Autodesk Inventor part; units mm, degrees
ref_plane "YZ Plane" through (0, 0, 0) normal (1, 0, 0) x (0, 1, 0)
ref_plane "XZ Plane" through (0, 0, 0) normal (0, 1, 0) x (-1, 0, 0)
ref_plane "XY Plane" through (0, 0, 0) normal (0, 0, 1) x (1, 0, 0)
sketch "Sketch1" plane through (0, 0, 0) normal (0, 1, 0) x (-1, 0, 0)
  line L0 (29.75, 29.75) -> (-29.75, 29.75)
  line L1 (-29.75, 29.75) -> (-29.75, -29.75)
  line L2 (-29.75, -29.75) -> (29.75, -29.75)
  line L3 (29.75, -29.75) -> (29.75, 29.75)
  line L4 (29.75, 0) -> (-29.75, 0) construction
  line L5 (0, -29.75) -> (0, 29.75) construction
  circle A0 centre (-22.75, 22.75) radius 1.75
  circle A1 centre (-22.75, -22.75) radius 1.75
  circle A2 centre (22.75, -22.75) radius 1.75
  circle A3 centre (22.75, 22.75) radius 1.75
  circle A4 centre (-1, 0) radius 0.25
  circle A5 centre (1, 0) radius 0.25
  point P0 (0, 0)
  dimension "d0" = 59.5
  dimension "d3" = 3.5
  dimension "d4" = 7
  dimension "d5" = 7
  dimension "d10" = 1
  dimension "d11" = 0.5
extrude "Extrusion1" add sketch "Sketch1" along normal blind 5
sketch "Sketch3" plane through (0, 5, 0) normal (0, 1, 0) x (1, 0, 0)
  circle A0 centre (0, 0) radius 24.25
  circle A1 centre (0, 0) radius 21.25
  line L0 (29.75, 29.75) -> (-29.75, 29.75)
  dimension "d7" = 3
  dimension "d12" = 5.5
extrude "Extrusion2" add sketch "Sketch3" along normal blind 4
properties part number "Power_Meter_Adapter_Part2"
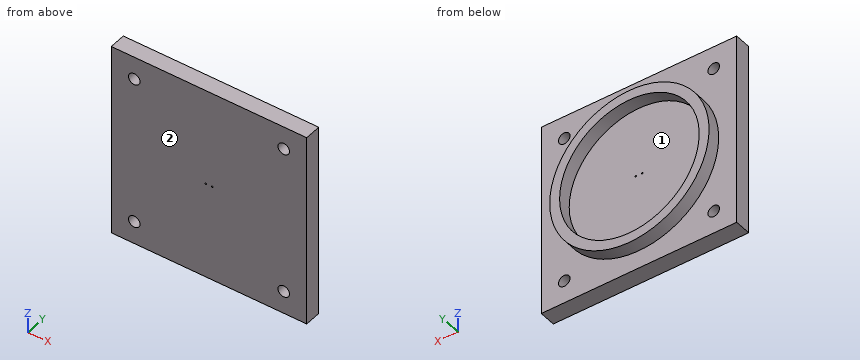
Check sheet for the modelled part. Datum: model origin and axes. Units: mm. Face numbers are marked on the shaded views. Coordinates: 2 decimals unless noted, no trailing zeros. Write each loop counter-clockwise with the first axis right and the second up, starting at its lowest first coordinate (ties: lowest second). Pieces come first, ordered by that corner, then holes.
Item 1: Mould release check, pull along Z, two halves, no side actions. Record for the marked faces 1 and 2: released by +Z, released by -Z, zero draft, split by the parting line, or undercut.
Numbers:
face 1: undercut
face 2: zero draft
Item 2: Cross-section at C-C on x = -23. Record the boundary of the cut face in (y, z).
Numbers:
outline: (0, -29.75) - (5, -29.75) - (5, -24.48) - (0, -24.48) - close; (0, -21.02) - (5, -21.02) - (5, -7.69) - (9, -7.69) - (9, 7.69) - (5, 7.69) - (5, 21.02) - (0, 21.02) - close; (0, 24.48) - (5, 24.48) - (5, 29.75) - (0, 29.75) - close
Item 3: Cross-section at B-B on z = 22.75. Record the boundary of the cut face in (x, y), then the cut area to 3 significant figures.
Numbers:
outline: (-29.75, 0) - (-24.5, 0) - (-24.5, 5) - (-29.75, 5) - close; (-21, 0) - (21, 0) - (21, 5) - (8.4, 5) - (8.4, 9) - (-8.4, 9) - (-8.4, 5) - (-21, 5) - close; (24.5, 0) - (29.75, 0) - (29.75, 5) - (24.5, 5) - close
area: 330 mm2
Item 4: Cross-section at D-D on z = -4.5. Record the boundary of the cut face in (x, y).
Numbers:
outline: (-29.75, 0) - (29.75, 0) - (29.75, 5) - (23.83, 5) - (23.83, 9) - (20.77, 9) - (20.77, 5) - (-20.77, 5) - (-20.77, 9) - (-23.83, 9) - (-23.83, 5) - (-29.75, 5) - close
Item 5: Cross-section at A-A on x = 0. Record the boundary of the cut face in (y, z).
Numbers:
outline: (0, -29.75) - (5, -29.75) - (5, -24.25) - (9, -24.25) - (9, -21.25) - (5, -21.25) - (5, 21.25) - (9, 21.25) - (9, 24.25) - (5, 24.25) - (5, 29.75) - (0, 29.75) - close
Item 6: Scan lines: probe 1 along Z at (x, y) = (-22.75, 2.3); probe 2 along Z at (x, y) = (0, 6.9); probe 3 along Z at (x, y) = (1, 1.95). Record each from-to range of solid material in increasing order.
Numbers:
probe 1: z = -29.75 to -24.5, -21 to 21, 24.5 to 29.75
probe 2: z = -24.25 to -21.25, 21.25 to 24.25
probe 3: z = -29.75 to -0.25, 0.25 to 29.75
Item 7: Depth check by flat-ended pin: pin 1 Ø1 at (x, y) = (-4, 7.5) entering from -Z; pin 2 Ø18 at (x, z) = (1, 1) entering from +Y. Enter the tip coordinate at first touch or a pass-through.
Numbers:
pin 1: stops at z = -24
pin 2: stops at y = 5
